CAD build for the part. Positions are in the model's coordinates, mm. A direction names the side the tool comes from. Round coordinates to 2 decimals unless told otherwise and drop trailing zeros. Order: outer loops, then holes, each group sorted by start corner. A loop starts at its lowest first (then second) coordinate and runs counter-clockwise, first axis right, second up. Notation, with made-up numbers: (-16.5, 8) -> (26.5, 8) arc R20 ccw to (26.5, 35) -> close; hole circle Ø9 at (47, 79.25). An arc over 180 degrees is marked (long way). Answer as CSV lines item,"result". Start each with the question number.
from build123d import *

# Parameters (mm, degrees)
SKETCH1_W           = 63
SKETCH1_H           = 126
BOSS_EXTRUDE1_DEPTH = 52
SKETCH2_W           = 63
SKETCH2_H           = 126
BOSS_EXTRUDE2_DEPTH = 2.5
SKETCH4_W           = 22.5
SKETCH4_H           = 32.5
CUT_EXTRUDE1_DEPTH  = 10
SKETCH5_W           = 22.5
SKETCH5_H           = 32.5
BOSS_EXTRUDE3_DEPTH = 1
SKETCH7_W           = 10
SKETCH7_H           = 32.5
BOSS_EXTRUDE6_DEPTH = 1
SKETCH8_W           = 11.6
SKETCH8_H           = 18.4
CUT_EXTRUDE2_DEPTH  = 90.058969228
SKETCH9_W           = 25
SKETCH9_H           = 25
CUT_EXTRUDE3_DEPTH  = 11
SKETCH10_W          = 24.67160759
SKETCH10_H          = 2
CUT_EXTRUDE4_DEPTH  = 11


with BuildPart() as part:
    # Sketch1 → Boss-Extrude1 (new body)
    with BuildSketch(Plane.XY):
        Rectangle(SKETCH1_W, SKETCH1_H)
        with BuildLine():
            Line((-27.55, 60.5), (27.55, 60.5))
            ThreePointArc((27.55, 60.5), (29, 61.95), (30.45, 60.5))
            ThreePointArc((30.45, 60.5), (30.025304833, 59.474695167), (29, 59.05))
            Line((29, 59.05), (29, -59.05))
            ThreePointArc((29, -59.05), (30.025304833, -59.474695167), (30.45, -60.5))
            ThreePointArc((30.45, -60.5), (29, -61.95), (27.55, -60.5))
            Line((27.55, -60.5), (-27.55, -60.5))
            ThreePointArc((-27.55, -60.5), (-30.025304833, -61.525304833), (-29, -59.05))
            Line((-29, -59.05), (-29, 59.05))
            ThreePointArc((-29, 59.05), (-30.025304833, 61.525304833), (-27.55, 60.5))
        make_face(mode=Mode.SUBTRACT)
    extrude(amount=BOSS_EXTRUDE1_DEPTH)

    # Sketch2 → Boss-Extrude2 (add)
    with BuildSketch(Plane(origin=(0, 0, 0), x_dir=(-1, 0, 0), z_dir=(0, 0, -1))):
        Rectangle(SKETCH2_W, SKETCH2_H)
    extrude(amount=BOSS_EXTRUDE2_DEPTH)

    # Sketch4 → Cut-Extrude1 (cut)
    with BuildSketch(Plane(origin=(0, 0, -2.5), x_dir=(-1, 0, 0), z_dir=(0, 0, -1))):
        with Locations((20.25, -46.75)):
            Rectangle(SKETCH4_W, SKETCH4_H)
    extrude(amount=-CUT_EXTRUDE1_DEPTH, mode=Mode.SUBTRACT)

    # Sketch5 → Boss-Extrude3 (add)
    with BuildSketch(Plane(origin=(0, 0, 7.5), x_dir=(-1, 0, 0), z_dir=(0, 0, -1))):
        with Locations((20.25, -46.75)):
            Rectangle(SKETCH5_W, SKETCH5_H)
    extrude(amount=-BOSS_EXTRUDE3_DEPTH)

    # Sketch7 → Boss-Extrude6 (add)
    with BuildSketch(Plane.ZY.offset(9)):
        with Locations((2.5, -46.75)):
            Rectangle(SKETCH7_W, SKETCH7_H)
    extrude(amount=BOSS_EXTRUDE6_DEPTH)

    # Sketch8 → Cut-Extrude2 (cut, through all)
    with BuildSketch(Plane(origin=(0, 0, -2.5), x_dir=(-1, 0, 0), z_dir=(0, 0, -1))):
        with Locations((16.2, 30)):
            Rectangle(SKETCH8_W, SKETCH8_H)
    extrude(amount=-CUT_EXTRUDE2_DEPTH, mode=Mode.SUBTRACT)

    # Sketch9 → Cut-Extrude3 (cut)
    with BuildSketch(Plane(origin=(0, 63, 0), x_dir=(1, 0, 0), z_dir=(0, 1, 0))):
        with Locations((-15.5, -19)):
            Rectangle(SKETCH9_W, SKETCH9_H)
    extrude(amount=-CUT_EXTRUDE3_DEPTH, mode=Mode.SUBTRACT)

    # Sketch10 → Cut-Extrude4 (cut)
    with BuildSketch(Plane(origin=(0, 63, 0), x_dir=(1, 0, 0), z_dir=(0, 1, 0))):
        with Locations((14.25, -7.5)):
            Rectangle(SKETCH10_W, SKETCH10_H)
        with Locations((14.25, -5.5)):
            Rectangle(SKETCH10_W, SKETCH10_H)
    extrude(amount=-CUT_EXTRUDE4_DEPTH, mode=Mode.SUBTRACT)


solid = part.part
Item 1: Band-saw the part on A-A, the plane y = 25. Give the cut face in (x, z).
Item 2: Mould opens along Y. For faces 4 (the flat face through (29, 1, 26)), 5 (the flat face through (26.586, 62, 7)), 6 (the flat face through (7, 63, 25)) say: released by +Y, released by -Y, zero draft, split by the parting line, or undercut.
Item 3: Band-saw the part on D-D, the plane x = -23.5. Give the cut face in (y, z).
Item 4: Probe line 1 (X direction, y = 55, z = 27.5); line 2 (Y direction, x = -2.5, z = 42.5); line 3 (Z direction, x = 19, y = 17). List the from-to ranges inside material, lowest first.
Item 5: Band-saw the part on B-B, the plane x = 21. Give the cut face in (y, z).
Item 6: Tool access for faces 1 (the flat face through (14, 62, 4.5)), 2 (the flat face through (-16, 20.8, -1)), 3 (the cylindrical face through (-30.06, 61.49, 25.64)): list every direction of +Z, -Z, +X, -X, +Y, -Y with a clear straight run to the whole face (end or side of a thin tool).
Item 7: Band-saw the part on C-C, the plane x = -14. Give the cut face in (y, z).
Item 8: Pin check, flat tips, straight feed: pin 1 (3 mm diameter, centred on x = -25.5, z = 3, fed in from -Y); pin 2 (5 mm diameter, centred on x = 12, y = 22.5, fed in from +Z); pin 3 (2.5 mm diameter, centred on x = -29, y = -60.5, fed in from +Z). Stop position of each tip, or through.
Values:
1,outline,"(-31.5, -2.5) -> (-22, -2.5) -> (-22, 0) -> (-29, 0) -> (-29, 52) -> (-31.5, 52) -> close; (-10.4, -2.5) -> (31.5, -2.5) -> (31.5, 52) -> (29, 52) -> (29, 0) -> (-10.4, 0) -> close"
2,face 4,"undercut"
2,face 5,"zero draft"
2,face 6,"released by +Y"
3,outline,"(-63, 7.5) -> (-30.5, 7.5) -> (-30.5, 8.5) -> (-60.5, 8.5) -> (-60.5, 52) -> (-63, 52) -> close; (-30.5, -2.5) -> (63, -2.5) -> (63, 6.5) -> (60.5, 6.5) -> (60.5, 0) -> (-30.5, 0) -> close; (60.5, 31.5) -> (63, 31.5) -> (63, 52) -> (60.5, 52) -> close"
4,line 1,"-31.5 to -29, 29 to 31.5"
4,line 2,"-63 to -60.5, 60.5 to 63"
4,line 3,"-2.5 to 0"
5,outline,"(-63, -2.5) -> (63, -2.5) -> (63, 4.5) -> (60.5, 4.5) -> (60.5, 0) -> (-60.5, 0) -> (-60.5, 52) -> (-63, 52) -> close; (60.5, 8.5) -> (63, 8.5) -> (63, 52) -> (60.5, 52) -> close"
6,face 1,"+Y"
6,face 2,"+Z, -Z"
6,face 3,"+Z"
7,outline,"(-63, 7.5) -> (-30.5, 7.5) -> (-30.5, 8.5) -> (-60.5, 8.5) -> (-60.5, 52) -> (-63, 52) -> close; (-30.5, -2.5) -> (20.8, -2.5) -> (20.8, 0) -> (-30.5, 0) -> close; (39.2, -2.5) -> (63, -2.5) -> (63, 6.5) -> (60.5, 6.5) -> (60.5, 0) -> (39.2, 0) -> close; (60.5, 31.5) -> (63, 31.5) -> (63, 52) -> (60.5, 52) -> close"
8,pin 1,"y = 60.5"
8,pin 2,"z = 0"
8,pin 3,"z = 8.5"
